```python
from build123d import *

# Parameters (mm, degrees)
SKETCH1_R               = 10
BOSS_EXTRUDE1_DEPTH     = 200
SKETCH2_R               = 20
BOSS_EXTRUDE2_DEPTH     = 20
SKETCH3_R               = 0.65
CUT_EXTRUDE1_DEPTH      = 5
SKETCH4_R               = 0.780836735
SKETCH4_R_2             = 0.65
CUT_EXTRUDE2_DEPTH      = 10
CUT_EXTRUDE3_DEPTH      = 202.990098767
CUT_EXTRUDE3_DEPTH_BACK = 202.990098767
SKETCH5_R               = 3


with BuildPart() as part:
    # Sketch1 → Boss-Extrude1 (new body)
    with BuildSketch(Plane.XY):
        Circle(SKETCH1_R)
    extrude(amount=BOSS_EXTRUDE1_DEPTH)

    # Sketch2 → Boss-Extrude2 (add)
    with BuildSketch(Plane.XY.offset(200)):
        Circle(SKETCH2_R)
    extrude(amount=-BOSS_EXTRUDE2_DEPTH)

    # Sketch3 → Cut-Extrude1 (cut)
    with BuildSketch(Plane.XY.offset(200)):
        with BuildLine():
            Line((0.398188886, 5.986772554), (-10.143967994, 13.726167778))
            ThreePointArc((-10.143967994, 13.726167778), (-13.384557042, 13.485311742), (-13.649708618, 10.246620085))
            Line((-13.649708618, 10.246620085), (-5.989590361, -0.353280782))
            ThreePointArc((-5.989590361, -0.353280782), (-4.258519498, -4.226702224), (-0.398188886, -5.986772554))
            Line((-0.398188886, -5.986772554), (10.143967994, -13.726167778))
            ThreePointArc((10.143967994, -13.726167778), (13.384557042, -13.485311742), (13.649708618, -10.246620085))
            Line((13.649708618, -10.246620085), (5.989590361, 0.353280782))
            ThreePointArc((5.989590361, 0.353280782), (4.258519498, 4.226702224), (0.398188886, 5.986772554))
        make_face()
        with Locations((11.623431116, -11.710928618)):
            Circle(SKETCH3_R, mode=Mode.SUBTRACT)
        with Locations((9.510080004, -9.581668869)):
            Circle(SKETCH3_R, mode=Mode.SUBTRACT)
        with Locations((-9.510080004, 9.581668869)):
            Circle(SKETCH3_R, mode=Mode.SUBTRACT)
        with Locations((-11.623431116, 11.710928618)):
            Circle(SKETCH3_R, mode=Mode.SUBTRACT)
    extrude(amount=-CUT_EXTRUDE1_DEPTH, mode=Mode.SUBTRACT)

    # Sketch4 → Cut-Extrude2 (cut)
    with BuildSketch(Plane.XY.offset(200)):
        with Locations((-9.510080004, 9.581668869)):
            Circle(SKETCH4_R)
        with Locations((-11.623431116, 11.710928618)):
            Circle(SKETCH4_R_2)
        with Locations((9.510080004, -9.581668869)):
            Circle(SKETCH4_R_2)
        with Locations((11.623431116, -11.710928618)):
            Circle(SKETCH4_R_2)
    extrude(amount=-CUT_EXTRUDE2_DEPTH, mode=Mode.SUBTRACT)

    # Sketch5 → Cut-Extrude3 (cut, two sides: drawn at the far end of the back side and taken through both)
    with BuildSketch(Plane(origin=(0, 0, 0), x_dir=(1, 0, 0), z_dir=(0, 1, 0)).offset(-CUT_EXTRUDE3_DEPTH_BACK)):
        with Locations(Location((0, -10, 0), (0, 0, 270))):
            Circle(SKETCH5_R)
    extrude(amount=CUT_EXTRUDE3_DEPTH + CUT_EXTRUDE3_DEPTH_BACK, mode=Mode.SUBTRACT)


solid = part.part
```
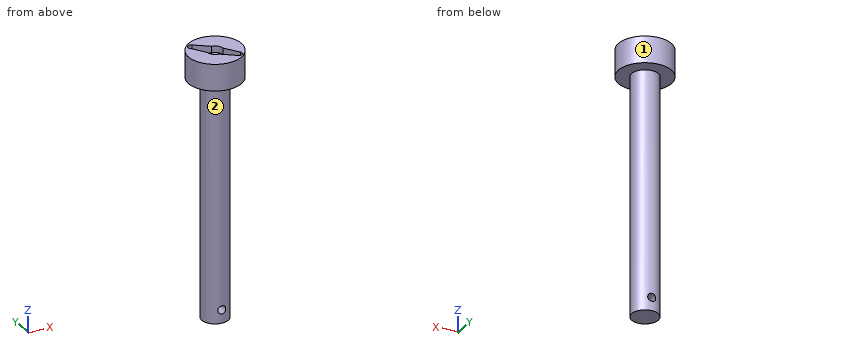
The listing builds one solid part. Answer for the finished solid, in the listing's coordinates (mm). Face numbers are marked on the shaded views. A direction names the side the tool comes from. Give positions to 0.01 mm unless a question says otherwise; leave off trailing zeros. Order: outer loops, then holes, each group sorted by start corner. A loop starts at its lowest first (then second) coordinate and runs counter-clockwise, first axis right, second up.
1) Find section B-B on z = 108. Write down the section's boundary in (x, y).
Reported:
outline: circle Ø20 at (0, 0)
2) For the marked faces 1 and 2, determine the directions among +Z, -Z, +X, -X, +Y, -Y from which every point of the face is accessible in a straight line to the end or side of a thin tool.
Reported:
face 1: +Z, -Z
face 2: -Z
3) Consider line 1 along Z through (x, y) = (0, 2); line 2 along Z through (x, y) = (14, -1.5); line 3 along Y through (x, z) = (-8, 53). Determine where each line is inside the solid, lowest interval first.
Reported:
line 1: z = 0 to 7, 13 to 195
line 2: z = 180 to 200
line 3: y = -6 to 6
4) Find section D-D on x = 17.5. Write down the section's boundary in (y, z), then the cut area to 3 significant figures.
Reported:
outline: (-9.68, 180) - (9.68, 180) - (9.68, 200) - (-9.68, 200) - close
area: 387 mm2
5) Find section A-A on y = 3.5. Write down the section's boundary in (x, z).
Reported:
outline: (-19.69, 180) - (-9.37, 180) - (-9.37, 0) - (9.37, 0) - (9.37, 180) - (19.69, 180) - (19.69, 200) - (4.87, 200) - (4.87, 195) - (-8.77, 195) - (-8.77, 200) - (-19.69, 200) - close; hole circle Ø6 at (0, 10)
6) Given P1, Ø5, axis at y = -2.5, z = 76.5, coming from the +X side; P2, Ø1.5, axis at x = -6, z = 125.5, coming from the -Y side; P3, Ø1.2, axis at x = -11.62, y = 11.71, coming from the +Z side, each flat-ended and moving along its own axis, determine where each tip first touches the part or whether it passes through.
Reported:
P1: stops at x = 10
P2: stops at y = -8.51
P3: stops at z = 190
7) Find section C-C on z = 10. Write down the section's boundary in (x, y).
Reported:
outline: (-3, -9.54) - (-3, 9.54) arc R10 ccw to start; (3, -9.54) arc R10 ccw to (3, 9.54) - close
